Build history of the part. All positions in model axes, mm. A direction names the side the tool comes from. Give positions to 0.01 mm unless a question says otherwise; leave off trailing zeros. Loops run counter-clockwise (first coordinate to the right, second up) from the corner with the lowest first, then second, coordinate; pieces in that order, holes last. Notation, with made-up numbers: M 65.25,36 L 76.25,36 A7 cw 76.25,42 Z; hole C 38.25,23 d3. An arc over 180 degrees is marked long. Answer in a Markdown table with one row per item. Add a question column.
```python
from build123d import *

# Parameters (mm, degrees)
SKETCH_5_R          = 3
EXTRUDE_1_DEPTH     = 3
CUT_EXTRUDE_1_DEPTH = 2
SKETCH_7_R          = 1.5
EXTRUDE_2_DEPTH     = 35


with BuildPart() as part:
    # ｽｹｯﾁ5 → ﾎﾞｽ - 押し出し1 (new body)
    with BuildSketch(Plane.XY):
        Circle(SKETCH_5_R)
    extrude(amount=EXTRUDE_1_DEPTH)

    # ｽｹｯﾁ6 → ｶｯﾄ - 押し出し1 (cut)
    with BuildSketch(Plane.XY.offset(3)):
        Polygon((1.443375673, 0), (0.721687836, 1.25), (-0.721687836, 1.25), (-1.443375673, 0), (-0.721687836, -1.25), (0.721687836, -1.25), align=None)
    extrude(amount=-CUT_EXTRUDE_1_DEPTH, mode=Mode.SUBTRACT)

    # ｽｹｯﾁ7 → ﾎﾞｽ - 押し出し2 (add)
    with BuildSketch(Plane(origin=(0, 0, 0), x_dir=(-1, 0, 0), z_dir=(0, 0, -1))):
        Circle(SKETCH_7_R)
    extrude(amount=EXTRUDE_2_DEPTH)


solid = part.part
```
(1) Slice it at B-B, the plane z = -17. Give the cut face in (x, y), then the cut area to 3 significant figures.
(2) Slice it at A-A, the plane x = 0. Give the cut face in (y, z), then the cut area to 3 significant figures.
(3) Wall check: line 1 (Z direction, x = -2.45, y = -1.6); line 2 (Y direction, x = -0.1, z = -28); line 3 (Z direction, x = -0.55, y = 0.7). Give the ranges that are in metal, low to high.
(4) Slice it at C-C, the plane y = -2.35. Give the cut face in (x, z), then the cut area to 3 significant figures.
(5) Slice it at D-D, the plane x = -2. Give the cut face in (y, z).
(6) Tool access for faces 1 (the flat face through (1.08, -0.63, 2.01)), 2 (the cylindrical face through (1.5, 0.07, -17.26)), 3 (the flat face through (1.3, -0.6, 3)): list every direction of +Z, -Z, +X, -X, +Y, -Y with a clear straight run to the whole face (end or side of a thin tool).
(7) Pull direction X, two halves, no side cores. Call faces 4 (the flat face through (0, -1.25, 2)), 5 (the cylindrical face through (-3, 0, 1)), 6 (the flat face through (0, 0, -35)), 7 (the flat face through (0, 0, 1)): +X half, -X half, draft (parallel to the pull), parting line (faces both ways), or undercut.
(8) Pin check, flat tips, straight feed: pin 1 (2 mm diameter, centred on x = 1, y = -2, fed in from -Z); pin 2 (1.5 mm diameter, centred on y = -0.5, z = -24, fed in from -X); pin 3 (1.2 mm diameter, centred on x = -0.5, y = 0, fed in from +Z). Stop position of each tip, or through.
Solution:
| question | item | result |
|---|---|---|
| 1 | outline | C 0,0 d3 |
| 1 | area | 7.07 mm^2 |
| 2 | outline | M -3,0 L -1.5,0 L -1.5,-35 L 1.5,-35 L 1.5,0 L 3,0 L 3,3 L 1.25,3 L 1.25,1 L -1.25,1 L -1.25,3 L -3,3 Z |
| 2 | area | 118 mm^2 |
| 3 | line 1 | 0 to 3 |
| 3 | line 2 | -1.5 to 1.5 |
| 3 | line 3 | -35 to 1 |
| 4 | outline | M -1.86,0 L 1.86,0 L 1.86,3 L -1.86,3 Z |
| 4 | area | 11.2 mm^2 |
| 5 | outline | M -2.24,0 L 2.24,0 L 2.24,3 L -2.24,3 Z |
| 6 | face 1 | +Z |
| 6 | face 2 | -Z |
| 6 | face 3 | +Z, +X, -X, +Y, -Y |
| 7 | face 4 | undercut |
| 7 | face 5 | parting line |
| 7 | face 6 | draft |
| 7 | face 7 | undercut |
| 8 | pin 1 | z = -35 |
| 8 | pin 2 | x = -1.5 |
| 8 | pin 3 | z = 1 |
